Can you work these out from the model? Positions are in its coordinate system, mm. Face numbers are marked on the shaded views. A direction names the side the tool comes from. Give positions to 0.01 mm unless a question says otherwise; leave off trailing zeros. Write each loop counter-clockwise with the first axis right and the second up, starting at its lowest first coordinate (ties: lowest second). Pieces come first, ordered by that corner, then holes. Notation, with made-up numbers: (30, -8) - (38, -8) arc R34 cw to (38, 31) - close; hole circle Ø3 at (66, 54.25). An arc over 180 degrees is marked (long way). Use a Markdown table: item, result. Add a question column.
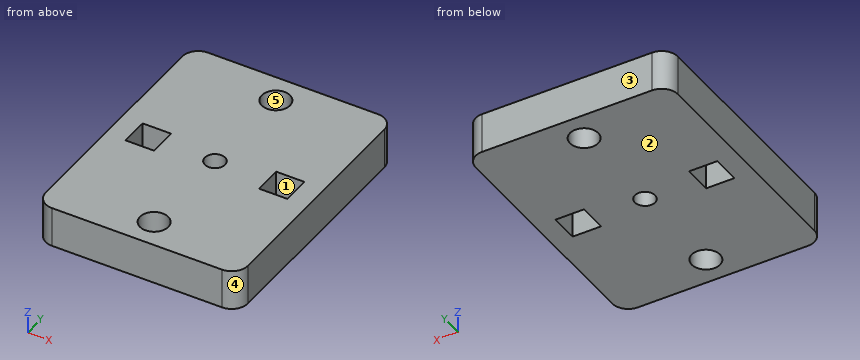
Autodesk Inventor part; units mm, degrees
ref_plane "YZ Plane" through (0, 0, 0) normal (1, 0, 0) x (0, 1, 0)
ref_plane "XZ Plane" through (0, 0, 0) normal (0, 1, 0) x (-1, 0, 0)
ref_plane "XY Plane" through (0, 0, 0) normal (0, 0, 1) x (1, 0, 0)
sketch "Skizze1" plane through (0, 0, 0) normal (0, 0, 1) x (1, 0, 0)
  line L0 (-18.0799, 0) -> (18.0799, 0)
  line L1 (0, -22.9799) -> (0, 22.9799)
  line L2 (-10.5, -16) -> (10.5, -16)
  line L3 (12.5, -14) -> (12.5, 14)
  line L4 (10.5, 16) -> (-10.5, 16)
  line L5 (-12.5, 14) -> (-12.5, -14)
  line L6 (-12.5, -16) -> (12.5, 16) construction
  line L7 (12.5, -16) -> (-12.5, 16) construction
  arc A0 (-10.5, 16) -> (-12.5, 14) centre (-10.5, 14) ccw
  arc A1 (-12.5, -14) -> (-10.5, -16) centre (-10.5, -14) ccw
  arc A2 (10.5, -16) -> (12.5, -14) centre (10.5, -14) ccw
  arc A3 (12.5, 14) -> (10.5, 16) centre (10.5, 14) ccw
  point P0 (0, 0)
  dimension "d0" = 25
  dimension "d1" = 32
  dimension "d2" = 2
extrude "Extrusion1" add sketch "Skizze1" against normal blind 5
sketch "Skizze2" plane through (0, 0, 0) normal (0, 0, 1) x (1, 0, 0)
  line L0 (12.5, -14) -> (12.5, 14)
  arc A0 (12.5, 14) -> (10.5, 16) centre (10.5, 14) ccw
  line L1 (10.5, 16) -> (-10.5, 16)
  arc A1 (-10.5, 16) -> (-12.5, 14) centre (-10.5, 14) ccw
  line L2 (-12.5, 14) -> (-12.5, -14)
  arc A2 (-12.5, -14) -> (-10.5, -16) centre (-10.5, -14) ccw
  line L3 (-10.5, -16) -> (10.5, -16)
  arc A3 (10.5, -16) -> (12.5, -14) centre (10.5, -14) ccw
  line L4 (-18.0799, 0) -> (18.0799, 0)
  line L5 (0, -22.9799) -> (0, 22.9799)
  circle A4 centre (0, 12.5) radius 1.75
  circle A5 centre (0, -12.5) radius 1.75
  point P0 (0, 0)
  dimension "d5" = 3.5
  dimension "d6" = 3.5
  dimension "d7" = 25
  dimension "d8" = 3.5
extrude "Extrusion2" cut sketch "Skizze2" against normal blind 5 contours A5 L5 | L5 A5 | A4 L5 | L5 A4
sketch "Skizze3" plane through (0, 0, 0) normal (0, 0, 1) x (1, 0, 0)
  circle A0 centre (0, -12.5) radius 1.75
  circle A1 centre (0, 12.5) radius 1.75
  line L0 (12.5, -14) -> (12.5, 14)
  arc A2 (12.5, 14) -> (10.5, 16) centre (10.5, 14) ccw
  line L1 (10.5, 16) -> (-10.5, 16)
  arc A3 (-10.5, 16) -> (-12.5, 14) centre (-10.5, 14) ccw
  line L2 (-12.5, 14) -> (-12.5, -14)
  arc A4 (-12.5, -14) -> (-10.5, -16) centre (-10.5, -14) ccw
  line L3 (-10.5, -16) -> (10.5, -16)
  arc A5 (10.5, -16) -> (12.5, -14) centre (10.5, -14) ccw
  line L4 (-18.0799, 0) -> (18.0799, 0)
  line L5 (0, -22.9799) -> (0, 22.9799)
  line L6 (-10, 1.75) -> (-6.5, 1.75)
  line L7 (-6.5, 1.75) -> (-6.5, -1.75)
  line L8 (-6.5, -1.75) -> (-10, -1.75)
  line L9 (-10, -1.75) -> (-10, 1.75)
  line L10 (6.5, 1.75) -> (10, 1.75)
  line L11 (10, 1.75) -> (10, -1.75)
  line L12 (10, -1.75) -> (6.5, -1.75)
  line L13 (6.5, -1.75) -> (6.5, 1.75)
  point P0 (0, 0)
  dimension "d11" = 3.5
  dimension "d12" = 3.5
  dimension "d13" = 3.5
  dimension "d14" = 3.5
  dimension "d15" = 13
extrude "Extrusion3" cut sketch "Skizze3" against normal blind 5 contours L7 L8 L9 L4 | L4 L9 L6 L7 | L13 L10 L11 L4 | L4 L11 L12 L13
sketch "Skizze4" plane through (0, 0, 0) normal (0, 0, 1) x (1, 0, 0)
  line L0 (6.5, 1.75) -> (10, 1.75)
  line L1 (10, 1.75) -> (10, -1.75)
  line L2 (10, -1.75) -> (6.5, -1.75)
  line L3 (6.5, -1.75) -> (6.5, 1.75)
  line L4 (-10, 1.75) -> (-6.5, 1.75)
  line L5 (-6.5, 1.75) -> (-6.5, -1.75)
  line L6 (-6.5, -1.75) -> (-10, -1.75)
  line L7 (-10, -1.75) -> (-10, 1.75)
  circle A0 centre (0, -12.5) radius 1.75
  circle A1 centre (0, 12.5) radius 1.75
  line L8 (12.5, -14) -> (12.5, 14)
  arc A2 (12.5, 14) -> (10.5, 16) centre (10.5, 14) ccw
  line L9 (10.5, 16) -> (-10.5, 16)
  arc A3 (-10.5, 16) -> (-12.5, 14) centre (-10.5, 14) ccw
  line L10 (-12.5, 14) -> (-12.5, -14)
  arc A4 (-12.5, -14) -> (-10.5, -16) centre (-10.5, -14) ccw
  line L11 (-10.5, -16) -> (10.5, -16)
  arc A5 (10.5, -16) -> (12.5, -14) centre (10.5, -14) ccw
  line L12 (-18.0799, 0) -> (18.0799, 0)
  line L13 (0, -22.9799) -> (0, 22.9799)
  circle A6 centre (0, 0) radius 1.25
  dimension "d18" = 2.5
extrude "Extrusion4" cut sketch "Skizze4" against normal blind 5 contours A6 L13 L12 | L12 L13 A6 | L13 A6 L12 | L12 A6 L13
properties part number "I Rückwand Adapter" material "PBT-Kunststoff"
Q1. Suppose I cut it at C-C (y = -12.5). Please give me the cut outline in (x, z).
Q2. Suppose I cut it at D-D (x = -8). Please give me the cut outline in (y, z), and give its area (4 significant figures).
Q3. If I drill on probe 1 along Y at (x, z) = (0, -1.35); probe 2 along X at (y, z) = (-12.5, -3.1); probe 3 along X at (y, z) = (0, -1.2), over which ranges is the centre line in solid material (lowest first)? Write a range as [from, to].
Q4. If we mould it in two halves opening along X, with no side actions, what happens to the marked faces 3, 4 and 5? For each: released by +X, released by -X, zero draft, split by the parting line, or undercut.
Q5. On a 3-axis mill with a long thin cutter (end or side, diameter ignored), from which of +Z, -Z, +X, -X, +Y, -Y can I reach the whole of each face in a straight line? I mean the marked faces 1 and 2. Say none if no direction works.
Q6. I'm going to push a flat-ended pin straight in: P1, Ø8, axis at x = -8, y = 5.5, coming from the +Z side. Where does the tip first touch, or does it pass through?
Q7. Suppose I cut it at B-B (x = 0). Please give me the cut outline in (y, z).
Q8. Suppose I cut it at A-A (y = 0). Please give me the cut outline in (x, z), and give its area (3 significant figures).
Derived:
| question | item | result |
|---|---|---|
| 1 | outline | (-12.5, -5) - (-1.75, -5) - (-1.75, 0) - (-12.5, 0) - close; (1.75, -5) - (12.5, -5) - (12.5, 0) - (1.75, 0) - close |
| 2 | outline | (-16, -5) - (-1.75, -5) - (-1.75, 0) - (-16, 0) - close; (1.75, -5) - (16, -5) - (16, 0) - (1.75, 0) - close |
| 2 | area | 142.5 mm² |
| 3 | probe 1 | [-16, -14.25], [-10.75, -1.25], [1.25, 10.75], [14.25, 16] |
| 3 | probe 2 | [-12.5, -1.75], [1.75, 12.5] |
| 3 | probe 3 | [-12.5, -10], [-6.5, -1.25], [1.25, 6.5], [10, 12.5] |
| 4 | face 3 | zero draft |
| 4 | face 4 | released by +X |
| 4 | face 5 | undercut |
| 5 | face 1 | +Z, -Z |
| 5 | face 2 | -Z, +X, -X, +Y, -Y |
| 6 | P1 | z = 0 |
| 7 | outline | (-16, -5) - (-14.25, -5) - (-14.25, 0) - (-16, 0) - close; (-10.75, -5) - (-1.25, -5) - (-1.25, 0) - (-10.75, 0) - close; (1.25, -5) - (10.75, -5) - (10.75, 0) - (1.25, 0) - close; (14.25, -5) - (16, -5) - (16, 0) - (14.25, 0) - close |
| 8 | outline | (-12.5, -5) - (-10, -5) - (-10, 0) - (-12.5, 0) - close; (-6.5, -5) - (-1.25, -5) - (-1.25, 0) - (-6.5, 0) - close; (1.25, -5) - (6.5, -5) - (6.5, 0) - (1.25, 0) - close; (10, -5) - (12.5, -5) - (12.5, 0) - (10, 0) - close |
| 8 | area | 77.5 mm² |
